Work out the finished part from the listing and answer in its coordinate system (mm). Face numbers are marked on the shaded views. A direction names the side the tool comes from. Coordinates: 2 decimals unless noted, no trailing zeros. Loops run counter-clockwise (first coordinate to the right, second up) from the corner with the lowest first, then second, coordinate; pieces in that order, holes last. Notation, with made-up numbers: (56.5, 23) -> (88.5, 23) arc R20 ccw to (88.5, 36) -> close; hole circle Ø6 at (53.25, 44). An arc over 180 degrees is marked (long way). Use a Markdown table: item, result.
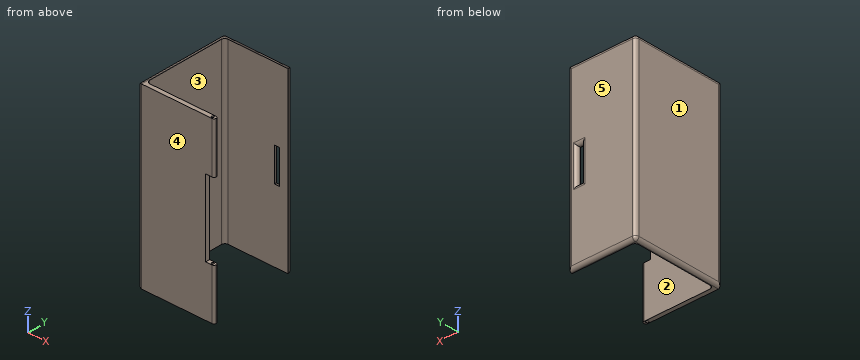
from build123d import *

# Parameters (mm, degrees)
F0_W      = 127
F0_H      = 266.7
F1_DEPTH  = 139.7
F2_T      = -6.35
F3_R      = 5.08
F4_DEPTH  = 25.4
F5_W      = 7.62
F5_H      = 50.8
F6_DEPTH  = 25.4
F7_R      = 1.905
F8_DEPTH  = 266.701
F9_R      = 5.08
F11_W     = 6.35
F11_H     = 76.2
F12_DEPTH = 12.7
F13_DEPTH = 266.701
F14_R     = 3.17499


# Not quite as in the source:
# - a fillet or chamfer is up to 0.001 mm smaller than in the source, because OpenCascade refuses the exact size


with BuildPart() as f1:
    # F0 (on Front) → F1 (new body)
    with BuildSketch(Plane.XZ):
        with Locations((-63.5, -133.35)):
            Rectangle(F0_W, F0_H)
    extrude(amount=F1_DEPTH)

    # F2
    f2_openings = [f1.faces().sort_by_distance(p)[0] for p in [
        (-63.5, -69.85, -266.7),
        (-63.5, -69.85, 0),
    ]]
    offset(amount=F2_T, openings=f2_openings)

    # F3
    f3_edges = [f1.edges().sort_by_distance(p)[0] for p in [
        (-6.35, -133.35, -133.35),
        (-120.65, -133.35, -133.35),
        (-6.35, -6.35, -133.35),
        (-120.65, -6.35, -133.35),
    ]]
    fillet(f3_edges, radius=F3_R)

    # F4 (cut): a face of the model
    f4_faces = [f1.faces().sort_by_distance(p)[0] for p in [
        (0, -69.85, -133.35),
    ]]
    extrude(f4_faces, amount=-F4_DEPTH, mode=Mode.SUBTRACT)

    # F5 (on face) → F6 (cut)
    with BuildSketch(Plane(origin=(0, 0, 0), x_dir=(-1, 0, 0), z_dir=(0, 1, 0))):
        with Locations((41.91, -133.35)):
            Rectangle(F5_W, F5_H)
    extrude(amount=-F6_DEPTH, mode=Mode.SUBTRACT)

    # F7 (on face) → F8 (cut, through all)
    with BuildSketch(Plane(origin=(0, 0, -266.7), x_dir=(1, 0, 0), z_dir=(0, 0, -1))):
        with Locations((-17.78, 136.525)):
            Circle(F7_R)
    extrude(amount=-F8_DEPTH, mode=Mode.SUBTRACT)

    # F9
    f9_edges = [f1.edges().sort_by_distance(p)[0] for p in [
        (-127, 0, -133.35),
        (-127, -69.85, -266.7),
        (-127, -69.85, 0),
        (-127, -139.7, -133.35),
        (-25.4, 0, -133.35),
        (-76.2, 0, -266.7),
        (-76.2, 0, 0),
        (-45.72, 0, -133.35),
        (-41.91, 0, -158.75),
        (-38.1, 0, -133.35),
        (-41.91, 0, -107.95),
    ]]
    fillet(f9_edges, radius=F9_R)

    # F11 (on offset) → F12 (join)
    with BuildSketch(Plane.YZ.offset(-25.4)):
        with Locations((-136.525, -38.1)):
            Rectangle(F11_W, F11_H)
        with Locations((-136.525, -228.6)):
            Rectangle(F11_W, F11_H)
    extrude(amount=F12_DEPTH)

    # F7 (on face) → F13 (cut, through all)
    with BuildSketch(Plane(origin=(0, 0, -266.7), x_dir=(1, 0, 0), z_dir=(0, 0, -1))):
        with Locations((-17.78, 136.525)):
            Circle(F7_R)
    extrude(amount=-F13_DEPTH, mode=Mode.SUBTRACT)

    # F14 (radius 3.175 in the source; OpenCascade refuses exactly that, so slightly less here)
    f14_edges = [f1.edges().sort_by_distance(p)[0] for p in [
        (-12.7, -133.35, -228.6),
        (-12.7, -133.35, -38.1),
        (-12.7, -139.7, -38.1),
        (-12.7, -139.7, -228.6),
    ]]
    fillet(f14_edges, radius=F14_R)


solid = f1.part
Q1. Determine the mould class of the marked faces 3, 4 and 5 for opening direction Y: pulls with the +Y half, pulls with the -Y half, needs draft (parallel to the pull), parting line crosses it, or undercut.
Solved:
| item | result |
|---|---|
| face 3 | undercut |
| face 4 | pulls with the -Y half |
| face 5 | pulls with the +Y half |
Q2. For the marked faces 1 and 2, determine the directions among +Z, -Z, +X, -X, +Y, -Y from which every point of the face is accessible in a straight line to the end or side of a thin tool.
Solved:
| item | result |
|---|---|
| face 1 | +Z, -Z, -X, +Y, -Y |
| face 2 | +Z, -Z, +X |
Q3. Consider line 1 (Y direction, x = -37, z = -213.5); line 2 (Y direction, x = -17.78, z = -208.5); line 3 (X direction, y = -128, z = -222). Determine where each line is inside the solid, lowest interval first. Write a range as [from, to].
Solved:
| item | result |
|---|---|
| line 1 | [-139.7, -133.35], [-6.35, 0] |
| line 2 | [-139.7, -138.43], [-134.62, -133.35] |
| line 3 | [-127, -120.65] |
Q4. Section D-D on z = -82 is taken. Determine the outline of the cut face in (x, y), and give its area (3 significant figures).
Solved:
| item | result |
|---|---|
| outline | (-127, -134.62) arc R5.08 ccw to (-121.92, -139.7) -> (-25.4, -139.7) -> (-25.4, -133.35) -> (-115.57, -133.35) arc R5.08 cw to (-120.65, -128.27) -> (-120.65, -11.43) arc R5.08 cw to (-115.57, -6.35) -> (-25.4, -6.35) -> (-25.4, -5.08) arc R5.08 ccw to (-30.48, 0) -> (-121.92, 0) arc R5.08 ccw to (-127, -5.08) -> close |
| area | 2,090 mm² |
Q5. Section C-C on y = -119.5 is taken. Determine the outline of the cut face in (x, z).
Solved:
| item | result |
|---|---|
| outline | (-127, -261.62) arc R5.08 ccw to (-121.92, -266.7) -> (-120.65, -266.7) -> (-120.65, 0) -> (-121.92, 0) arc R5.08 ccw to (-127, -5.08) -> close |
Q6. Section B-B on z = -126 is taken. Determine the outline of the cut face in (x, y), and give its area (3 significant figures).
Solved:
| item | result |
|---|---|
| outline | (-127, -134.62) arc R5.08 ccw to (-121.92, -139.7) -> (-25.4, -139.7) -> (-25.4, -133.35) -> (-115.57, -133.35) arc R5.08 cw to (-120.65, -128.27) -> (-120.65, -11.43) arc R5.08 cw to (-115.57, -6.35) -> (-45.72, -6.35) -> (-45.72, -5.08) arc R5.08 ccw to (-50.8, 0) -> (-121.92, 0) arc R5.08 ccw to (-127, -5.08) -> close; (-38.1, -6.35) -> (-25.4, -6.35) -> (-25.4, -5.08) arc R5.08 ccw to (-30.48, 0) -> (-33.02, 0) arc R5.08 ccw to (-38.1, -5.08) -> close |
| area | 2,030 mm² |
Q7. Given pin 1 Ø1.9 at (y, z) = (-135.5, -130.5) entering from +X; pin 2 Ø10 at (y, z) = (-25, -62.5) entering from +X, each flat-ended and moving along its own axis, determine where each tip first touches the part or whether it passes through.
Solved:
| item | result |
|---|---|
| pin 1 | x = -25.4 |
| pin 2 | x = -120.65 |
Q8. Section A-A on x = -108 is taken. Determine the outline of the cut face in (y, z), and give its area (3 significant figures).
Solved:
| item | result |
|---|---|
| outline | (-139.7, -266.7) -> (-133.35, -266.7) -> (-133.35, 0) -> (-139.7, 0) -> close; (-6.35, -266.7) -> (-5.08, -266.7) arc R5.08 ccw to (0, -261.62) -> (0, -5.08) arc R5.08 ccw to (-5.08, 0) -> (-6.35, 0) -> close |
| area | 3,380 mm² |
